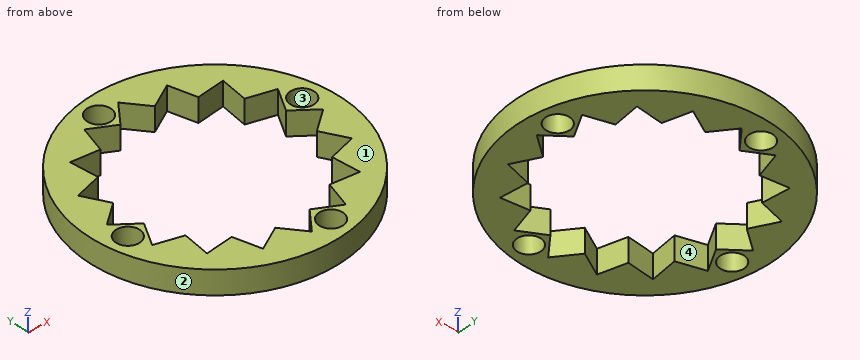
from build123d import *

# Parameters (mm, degrees)
ESBO_O1_R                = 32
ESBO_O1_R_2              = 27
RESSALTO_EXTRUS_O2_DEPTH = 6
ESBO_O3_R                = 3
CORTE_EXTRUS_O1_DEPTH    = 46.650848842
ESBO_O4_R                = 3
ESBO_O4_R_2              = 3.281084103
RESSALTO_EXTRUS_O3_DEPTH = 6


with BuildPart() as part:
    # Esboço1 → Ressalto-extrusão2 (new body)
    # profile 1 of 17: a face of its own
    with BuildSketch(Plane.XY):
        Circle(ESBO_O1_R)
        Circle(ESBO_O1_R_2, mode=Mode.SUBTRACT)
    # profile 2 of 17: a face of its own
    with BuildSketch(Plane.XY):
        with BuildLine():
            Line((-4.291987084, 21.577276169), (0, 27))
            ThreePointArc((0, 27), (-5.267438694, 26.481202571), (-10.332452674, 24.944747378))
            Line((-10.332452674, 24.944747378), (-4.291987084, 21.577276169))
        make_face()
    # profile 3 of 17: a face of its own
    with BuildSketch(Plane.XY):
        with BuildLine():
            Line((-12.222545126, 18.292331471), (-10.332452674, 24.944747378))
            ThreePointArc((-10.332452674, 24.944747378), (-15.000396292, 22.449679532), (-19.091883092, 19.091883092))
            Line((-19.091883092, 19.091883092), (-12.222545126, 18.292331471))
        make_face()
    # profile 4 of 17: a face of its own
    with BuildSketch(Plane.XY):
        with BuildLine():
            Line((-18.292331471, 12.222545126), (-19.091883092, 19.091883092))
            ThreePointArc((-19.091883092, 19.091883092), (-22.449679532, 15.000396292), (-24.944747378, 10.332452674))
            Line((-24.944747378, 10.332452674), (-18.292331471, 12.222545126))
        make_face()
    # profile 5 of 17: a face of its own
    with BuildSketch(Plane.XY):
        with BuildLine():
            Line((-21.577276169, 4.291987084), (-24.944747378, 10.332452674))
            ThreePointArc((-24.944747378, 10.332452674), (-26.481202571, 5.267438694), (-27, 0))
            Line((-27, 0), (-21.577276169, 4.291987084))
        make_face()
    # profile 6 of 17: a face of its own
    with BuildSketch(Plane.XY):
        with BuildLine():
            Line((-21.577276169, -4.291987084), (-27, 0))
            ThreePointArc((-27, 0), (-26.481202571, -5.267438694), (-24.944747378, -10.332452674))
            Line((-24.944747378, -10.332452674), (-21.577276169, -4.291987084))
        make_face()
    # profile 7 of 17: a face of its own
    with BuildSketch(Plane.XY):
        with BuildLine():
            Line((-18.292331471, -12.222545126), (-24.944747378, -10.332452674))
            ThreePointArc((-24.944747378, -10.332452674), (-22.449679532, -15.000396292), (-19.091883092, -19.091883092))
            Line((-19.091883092, -19.091883092), (-18.292331471, -12.222545126))
        make_face()
    # profile 8 of 17: a face of its own
    with BuildSketch(Plane.XY):
        with BuildLine():
            Line((-12.222545126, -18.292331471), (-19.091883092, -19.091883092))
            ThreePointArc((-19.091883092, -19.091883092), (-15.000396292, -22.449679532), (-10.332452674, -24.944747378))
            Line((-10.332452674, -24.944747378), (-12.222545126, -18.292331471))
        make_face()
    # profile 9 of 17: a face of its own
    with BuildSketch(Plane.XY):
        with BuildLine():
            Line((-4.291987084, -21.577276169), (-10.332452674, -24.944747378))
            ThreePointArc((-10.332452674, -24.944747378), (-5.267438694, -26.481202571), (0, -27))
            Line((0, -27), (-4.291987084, -21.577276169))
        make_face()
    # profile 10 of 17: a face of its own
    with BuildSketch(Plane.XY):
        with BuildLine():
            ThreePointArc((0, -27), (5.267438694, -26.481202571), (10.332452674, -24.944747378))
            Line((10.332452674, -24.944747378), (4.291987084, -21.577276169))
            Line((4.291987084, -21.577276169), (0, -27))
        make_face()
    # profile 11 of 17: a face of its own
    with BuildSketch(Plane.XY):
        with BuildLine():
            ThreePointArc((10.332452674, -24.944747378), (15.000396292, -22.449679532), (19.091883092, -19.091883092))
            Line((19.091883092, -19.091883092), (12.222545126, -18.292331471))
            Line((12.222545126, -18.292331471), (10.332452674, -24.944747378))
        make_face()
    # profile 12 of 17: a face of its own
    with BuildSketch(Plane.XY):
        with BuildLine():
            ThreePointArc((19.091883092, -19.091883092), (22.449679532, -15.000396292), (24.944747378, -10.332452674))
            Line((24.944747378, -10.332452674), (18.292331471, -12.222545126))
            Line((18.292331471, -12.222545126), (19.091883092, -19.091883092))
        make_face()
    # profile 13 of 17: a face of its own
    with BuildSketch(Plane.XY):
        with BuildLine():
            ThreePointArc((24.944747378, -10.332452674), (26.481202571, -5.267438694), (27, 0))
            Line((27, 0), (21.577276169, -4.291987084))
            Line((21.577276169, -4.291987084), (24.944747378, -10.332452674))
        make_face()
    # profile 14 of 17: a face of its own
    with BuildSketch(Plane.XY):
        with BuildLine():
            ThreePointArc((27, 0), (26.481202571, 5.267438694), (24.944747378, 10.332452674))
            Line((24.944747378, 10.332452674), (21.577276169, 4.291987084))
            Line((21.577276169, 4.291987084), (27, 0))
        make_face()
    # profile 15 of 17: a face of its own
    with BuildSketch(Plane.XY):
        with BuildLine():
            ThreePointArc((24.944747378, 10.332452674), (22.449679532, 15.000396292), (19.091883092, 19.091883092))
            Line((19.091883092, 19.091883092), (18.292331471, 12.222545126))
            Line((18.292331471, 12.222545126), (24.944747378, 10.332452674))
        make_face()
    # profile 16 of 17: a face of its own
    with BuildSketch(Plane.XY):
        with BuildLine():
            ThreePointArc((19.091883092, 19.091883092), (15.000396292, 22.449679532), (10.332452674, 24.944747378))
            Line((10.332452674, 24.944747378), (12.222545126, 18.292331471))
            Line((12.222545126, 18.292331471), (19.091883092, 19.091883092))
        make_face()
    # profile 17 of 17: a face of its own
    with BuildSketch(Plane.XY):
        with BuildLine():
            ThreePointArc((10.332452674, 24.944747378), (5.267438694, 26.481202571), (0, 27))
            Line((0, 27), (4.291987084, 21.577276169))
            Line((4.291987084, 21.577276169), (10.332452674, 24.944747378))
        make_face()
    extrude(amount=RESSALTO_EXTRUS_O2_DEPTH)

    # Esboço3 → Corte-extrusão1 (cut, through all)
    with BuildSketch(Plane.XY.offset(6)):
        with Locations((-5.267438694, 26.481202571)):
            Circle(ESBO_O3_R)
        with Locations((5.267438694, -26.481202571)):
            Circle(ESBO_O3_R)
        with Locations((26.481202571, 5.267438694)):
            Circle(ESBO_O3_R)
        with Locations((-26.481202571, -5.267438694)):
            Circle(ESBO_O3_R)
        with Locations((22.449679532, -15.000396292)):
            Circle(ESBO_O3_R)
        with Locations((-22.449679532, 15.000396292)):
            Circle(ESBO_O3_R)
    extrude(amount=-CORTE_EXTRUS_O1_DEPTH, mode=Mode.SUBTRACT)

    # Esboço4 → Ressalto-extrusão3 (add)
    with BuildSketch(Plane.XY.offset(6)):
        with Locations((-22.449679532, 15.000396292)):
            Circle(ESBO_O4_R)
        with Locations((22.424396541, -15.280341006)):
            Circle(ESBO_O4_R_2)
    extrude(amount=-RESSALTO_EXTRUS_O3_DEPTH)


solid = part.part
Check sheet for the modelled part. Datum: model origin and axes. Units: mm. Face numbers are marked on the shaded views. Round coordinates to 2 decimals unless told otherwise and drop trailing zeros. Order: outer loops, then holes, each group sorted by start corner. A loop starts at its lowest first (then second) coordinate and runs counter-clockwise, first axis right, second up.
(1) Go/stop test with flat-tipped pins: P1, Ø1, axis at y = -2, z = 4.5, coming from the +X side; P2, Ø2, axis at x = -18.5, z = 4, coming from the +Y side; P3, Ø5, axis at x = -20, y = -15, coming from the -Z side. Record where each tip stops, or that it passes through.
(2) Cross-section at C-C, the plane z = 1.8. State how many separate pieces and enclosed holes the cut face has, and give its area (3 significant figures).
(3) Draft check along Y on the marked faces 1, 2, 3 and 4. Enter one of: pulls with the +Y half, pulls with the -Y half, needs draft (parallel to the pull), parting line crosses it, or undercut.
(4) Scan lines: probe 1 along X at (y, z) = (22.5, 1.5); probe 2 along Y at (x, z) = (-3, 2.55); probe 3 along Y at (x, z) = (-4.5, 3.3). Record each from-to range of solid material in increasing order.
(5) Cross-section at A-A, the plane y = -16.5. Enter the section's corners in (x, z).
(6) Cross-section at B-B, the plane x = -3.5. Enter the section's corners in (y, z).
Check sheet entries:
1. P1: stops at x = 31.96
1. P2: stops at y = 26.79
1. P3: stops at z = 0
2. separate pieces: 1
2. enclosed holes: 5
2. area: 1,250 mm2
3. face 1: needs draft
3. face 2: parting line crosses it
3. face 3: undercut
3. face 4: undercut
4. probe 1: x = -22.75 to -11.03, -5.95 to -3.56, 3.56 to 5.95, 11.03 to 22.75
4. probe 2: y = -31.86 to -23.21, 23.21 to 24.52, 28.45 to 31.86
4. probe 3: y = -31.68 to -21.69, 21.69 to 23.58, 29.38 to 31.68
5. outline: (-27.42, 0) - (-18.79, 0) - (-18.79, 6) - (-27.42, 6) - close; (18.79, 0) - (27.42, 0) - (27.42, 6) - (18.79, 6) - close
6. outline: (-31.81, 0) - (-22.58, 0) - (-22.58, 6) - (-31.81, 6) - close; (22.58, 0) - (24.06, 0) - (24.06, 6) - (22.58, 6) - close; (28.91, 0) - (31.81, 0) - (31.81, 6) - (28.91, 6) - close
